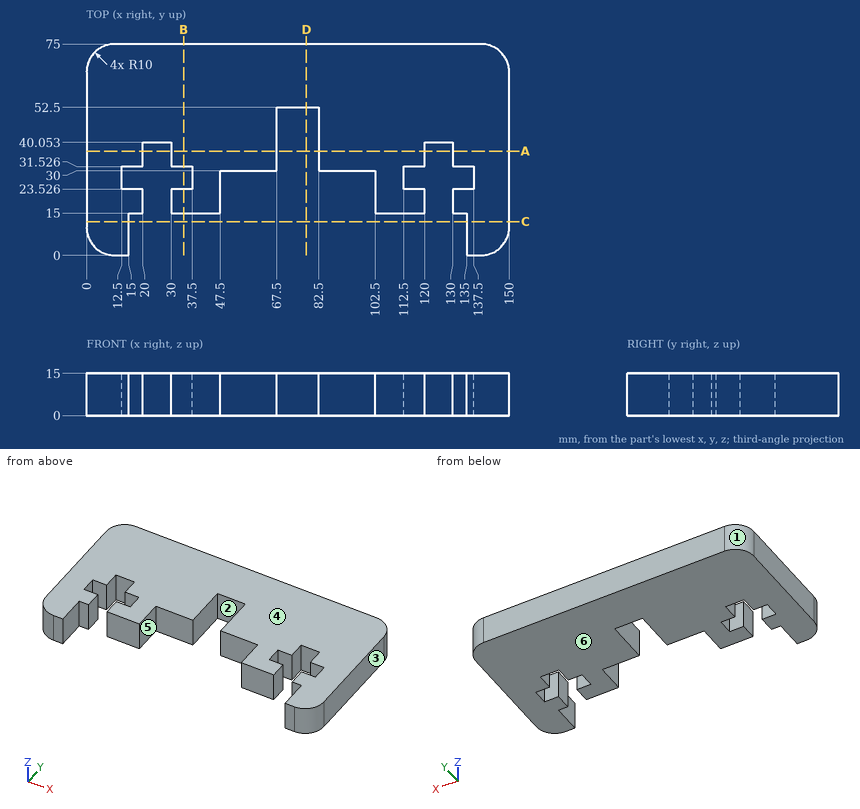
Geometry check sheet. Reference: drawing and pictorial views, mm from the part's lowest x, y, z. A direction names the side the tool comes from. Give positions to 0.01 mm unless a question says otherwise; leave off trailing zeros. Loops run counter-clockwise (first coordinate to the right, second up) from the corner with the lowest first, then second, coordinate; pieces in that order, holes last.
1. Section check A-A, the plane y = 37. Enter the section's corners in (x, z).
2. Mould release check, pull along X, two halves, no side actions. Record for the marked faces 1, 2, 3 and 4: released by +X, released by -X, zero draft, split by the parting line, or undercut.
3. Thickness scan on line 1 (X direction, y = 17.5, z = 8.75); line 2 (X direction, y = 25.5, z = 13.25); line 3 (X direction, y = 41.5, z = 7). Record the ranges inside material, lowest first.
4. Go/stop test with flat-tipped pins: pin 1 Ø7.5 at (x, z) = (54, 6) entering from -Y; pin 2 Ø1.5 at (x, y) = (120, 12.5) entering from -Z; pin 3 Ø4.5 at (x, z) = (72, 9) entering from -Y; pin 4 Ø4 at (x, z) = (34, 6.5) entering from -Y. Record where each tip stops, or that it passes through.
5. Section check D-D, the plane x = 78. Enter the section's corners in (y, z).
6. Section check B-B, the plane x = 34.5. Enter the section's corners in (y, z), then the cut area to 3 significant figures.
7. Section check C-C, the plane y = 12. Enter the section's corners in (x, z), then the cut area to 3 significant figures.
8. Set-up check for the marked faces 5 and 6: record each of +Z, -Z, +X, -X, +Y, -Y from which the full face is reachable in a straight line by a thin tool's end or side.
Geometry says:
1. outline: (0, 0) - (20, 0) - (20, 15) - (0, 15) - close; (30, 0) - (67.5, 0) - (67.5, 15) - (30, 15) - close; (82.5, 0) - (120, 0) - (120, 15) - (82.5, 15) - close; (130, 0) - (150, 0) - (150, 15) - (130, 15) - close
2. face 1: released by -X
2. face 2: undercut
2. face 3: released by +X
2. face 4: zero draft
3. line 1: x = 0 to 20, 30 to 47.5, 102.5 to 120, 130 to 150
3. line 2: x = 0 to 12.5, 37.5 to 47.5, 102.5 to 112.5, 137.5 to 150
3. line 3: x = 0 to 67.5, 82.5 to 150
4. pin 1: stops at y = 30
4. pin 2: passes through
4. pin 3: stops at y = 52.5
4. pin 4: stops at y = 15
5. outline: (52.5, 0) - (75, 0) - (75, 15) - (52.5, 15) - close
6. outline: (15, 0) - (23.53, 0) - (23.53, 15) - (15, 15) - close; (31.53, 0) - (75, 0) - (75, 15) - (31.53, 15) - close
6. area: 780 mm2
7. outline: (0, 0) - (15, 0) - (15, 15) - (0, 15) - close; (135, 0) - (150, 0) - (150, 15) - (135, 15) - close
7. area: 450 mm2
8. face 5: +Z, -Z, -Y
8. face 6: -Z, +X, -X, +Y, -Y
